Check sheet for the modelled part. Datum: model origin and axes. Units: mm. A direction names the side the tool comes from. Give positions to 0.01 mm unless a question says otherwise; leave off trailing zeros. Order: outer loops, then holes, each group sorted by start corner. A loop starts at its lowest first (then second) coordinate and runs counter-clockwise, first axis right, second up.
Item 1: Material ranges on line 1 along Z through (x, y) = (0.45, 28); line 2 along Z through (x, y) = (1.6, 25); line 3 along Y through (x, z) = (1.5, 3.5), recorded low to high.
Item 2: Sectioned sample at B-B on y = 24.84. Record the boundary of the cut face in (x, z).
Item 3: Sectioned sample at C-C on x = 1.4. Record the boundary of the cut face in (y, z).
Item 4: Sectioned sample at A-A on z = 19.5. Record the boundary of the cut face in (x, y), and give its area (3 significant figures).
Item 5: Access from +Z, -Z, +X, -X, +Y, -Y to the whole of each face (thin tool, end or side, straight path). Record for faces 1 (the flat face through (0, 44, 25)), 2 (the flat face through (1, 17, 0)), 3 (the flat face through (1.52, 63.18, 53.99)).
Item 6: Gauge pin test, flat ends, axial feed: P1, Ø1.5, axis at x = 1, y = 44, coming from the -Z side; P2, Ø0.9, axis at x = 1.5, y = 27, coming from the +Z side; P3, Ø8, axis at y = 55.5, z = 12.5, coming from the -X side; P4, Ø1.5, axis at x = 2, z = 43.5, coming from the +Y side. Record the tip position at first contact, or that the pin passes through.
Item 7: Release check for a two-part mould opening along Z. For faces 4 (the cylindrical face through (1.52, 3.77, 1.61)), 5 (the flat face through (1, 28.65, -1)), 6 (the flat face through (1, 42, 0)), 7 (the flat face through (2, 25, 2.54)) record: released by +Z, released by -Z, zero draft, split by the parting line, or undercut.
Item 8: Sectioned sample at D-D on y = 15.5. Record the boundary of the cut face in (x, z), and give its area (3 significant figures).
from build123d import *

# Parameters (mm, degrees)
F1_DEPTH = 3
F2_R     = 19.05
F3_R     = 2.54
F5_DEPTH = 3
F7_DEPTH = 3


with BuildPart() as f1:
    # F0 (on Right) → F1 (new body)
    with BuildSketch(Plane.YZ):
        with BuildLine():
            Line((70.710678, 70.710678), (0, 0))
            Line((0, 0), (28.65, 0))
            Line((28.65, 0), (28.65, -3))
            Line((28.65, -3), (41.35, -3))
            Line((41.35, -3), (41.35, 0))
            Line((41.35, 0), (56.030339, 0))
            ThreePointArc((56.030339, 0), (67.001876, 34.601426), (70.710678, 70.710678))
        make_face()
    extrude(amount=F1_DEPTH)

    # F2
    f2_edges = [f1.edges().sort_by_distance(p)[0] for p in [
        (1.5, 56.030339, 0),
    ]]
    fillet(f2_edges, radius=F2_R)

    # F3
    f3_edges = [f1.edges().sort_by_distance(p)[0] for p in [
        (1.5, 70.710678, 70.710678),
        (1.5, 0, 0),
    ]]
    fillet(f3_edges, radius=F3_R)

    # F4 (on face) → F5 (cut, through all)
    with BuildSketch(Plane.YZ.offset(3)):
        Polygon((30.257099, 25.307352), (21.276843, 16.327096), (23.398163, 14.205775), (32.37842, 23.186031), align=None)
        Polygon((65.612438, 60.662691), (56.632182, 51.682435), (58.753502, 49.561114), (67.733759, 58.54137), align=None)
    extrude(amount=-F5_DEPTH, mode=Mode.SUBTRACT)

    # F6 (on face) → F7 (cut, through all)
    with BuildSketch(Plane.YZ.offset(3)):
        with BuildLine():
            Line((14.68, 2.54), (35, 2.54))
            ThreePointArc((35, 2.54), (24.84, 12.7), (14.68, 2.54))
        make_face()
    extrude(amount=-F7_DEPTH, mode=Mode.SUBTRACT)


solid = f1.part
Report:
1. line 1: z = 0 to 2.54, 12.2 to 18.81, 23.05 to 28
1. line 2: z = 0 to 2.54, 12.7 to 15.81, 20.05 to 25
1. line 3: y = 3.78 to 14.73, 34.95 to 54.01
2. outline: (0, 0) - (3, 0) - (3, 2.54) - (0, 2.54) - close; (0, 12.7) - (3, 12.7) - (3, 15.65) - (0, 15.65) - close; (0, 19.89) - (3, 19.89) - (3, 24.84) - (0, 24.84) - close
3. outline: (4.34, 4.34) arc R2.54 ccw to (6.13, 0) - (28.65, 0) - (28.65, -3) - (41.35, -3) - (41.35, 0) - (43.01, 0) arc R19.05 ccw to (61.02, 12.84) arc R177.64 ccw to (70.6, 64.38) arc R2.54 ccw to (66.26, 66.26) - close; hole (14.68, 2.54) - (35, 2.54) arc R10.16 ccw to start; hole (21.28, 16.33) - (23.4, 14.21) - (32.38, 23.19) - (30.26, 25.31) - close; hole (56.63, 51.68) - (58.75, 49.56) - (67.73, 58.54) - (65.61, 60.66) - close
4. outline: (0, 19.5) - (3, 19.5) - (3, 24.45) - (0, 24.45) - close; (0, 28.69) - (3, 28.69) - (3, 63.17) - (0, 63.17) - close
4. area: 118 mm2
5. face 1: +Z, -Z, -X, +Y, -Y
5. face 2: -Z, +X, -X, -Y
5. face 3: +X, -X
6. P1: stops at z = 0
6. P2: stops at z = 27.45
6. P3: stops at x = 0
6. P4: stops at y = 68.73
7. face 4: split by the parting line
7. face 5: zero draft
7. face 6: released by -Z
7. face 7: undercut
8. outline: (0, 0) - (3, 0) - (3, 2.54) - (0, 2.54) - close; (0, 6.54) - (3, 6.54) - (3, 15.5) - (0, 15.5) - close
8. area: 34.5 mm2
